Print and shaded views of the part. All mm, measured from the part's lowest x, y and z. Round coordinates to 2 decimals unless told otherwise and drop trailing zeros. Order: outer loops, then holes, each group sorted by start corner. A loop starts at its lowest first (then second) coordinate and runs counter-clockwise, first axis right, second up.
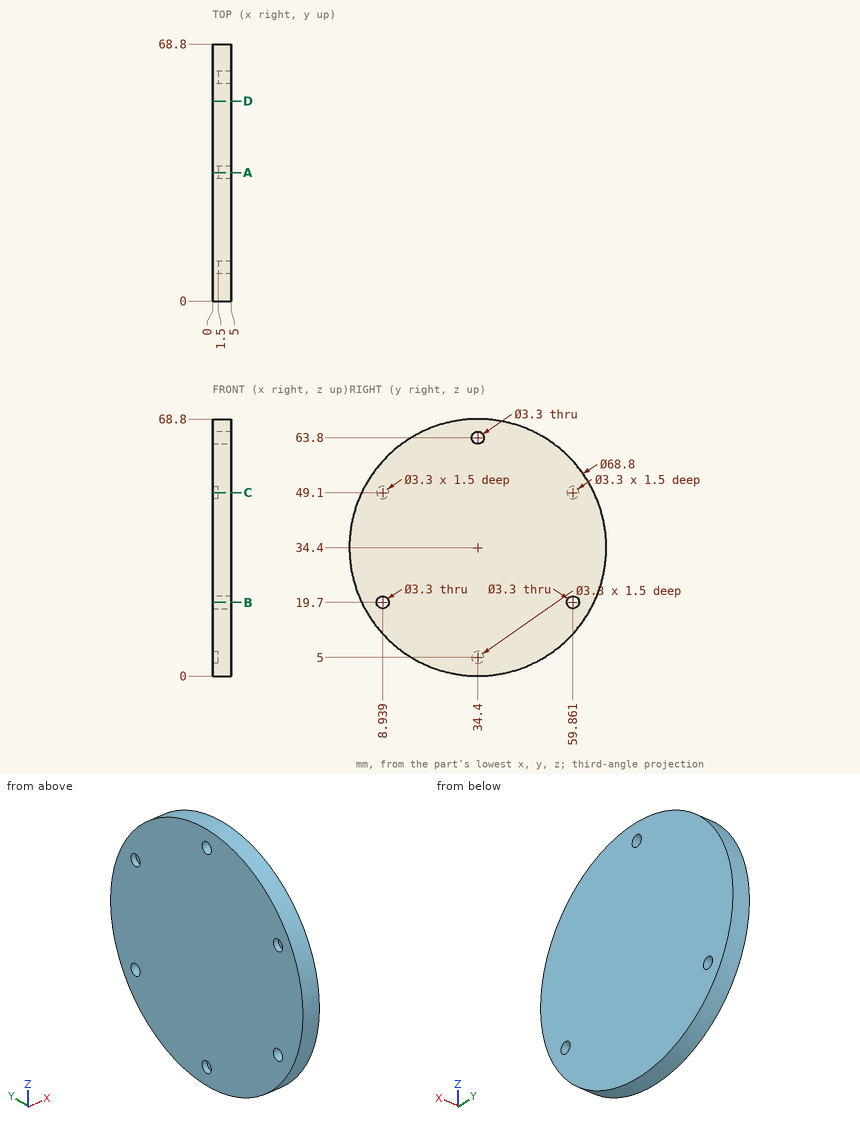
1. Pin check, flat tips, straight feed: P1, Ø1, axis at y = 9, z = 49, coming from the -X side; P2, Ø2, axis at x = 2.5, y = 56.5, coming from the -Z side; P3, Ø3, axis at x = 3, y = 31, coming from the +Z side. Stop position of each tip, or through.
2. Cut at B-B, the plane z = 19.7. Write the cut outline in (x, y), and give its area (3 significant figures).
3. Cut at A-A, the plane y = 34.4. Write the cut outline in (x, z).
4. Cut at C-C, the plane z = 49.1. Write the cut outline in (x, y).
5. Cut at D-D, the plane y = 53.5. Write the cut outline in (x, z).
6. Drill centre lines: line 1 (Y direction, x = 1.15, z = 49.1); line 2 (Y direction, x = 3.95, z = 64.5) (1 decimal); line 3 (Y direction, x = 4.7, z = 20.5). Where is each one in solid material? Low to high.
Outcome:
1. P1: stops at x = 1.5
1. P2: stops at z = 7.23
1. P3: stops at z = 68.75
2. outline: (0, 3.3) - (5, 3.3) - (5, 7.29) - (0, 7.29) - close; (0, 10.59) - (5, 10.59) - (5, 58.21) - (0, 58.21) - close; (0, 61.51) - (5, 61.51) - (5, 65.5) - (0, 65.5) - close
2. area: 278 mm2
3. outline: (0, 0) - (5, 0) - (5, 62.15) - (0, 62.15) - (0, 6.65) - (1.5, 6.65) - (1.5, 3.35) - (0, 3.35) - close; (0, 65.45) - (5, 65.45) - (5, 68.8) - (0, 68.8) - close
4. outline: (0, 3.3) - (5, 3.3) - (5, 65.5) - (0, 65.5) - (0, 61.51) - (1.5, 61.51) - (1.5, 58.21) - (0, 58.21) - (0, 10.59) - (1.5, 10.59) - (1.5, 7.29) - (0, 7.29) - close
5. outline: (0, 5.79) - (5, 5.79) - (5, 63.01) - (0, 63.01) - close
6. line 1: y = 3.3 to 7.29, 10.59 to 58.21, 61.51 to 65.5
6. line 2: y = 17.7 to 32.9, 35.9 to 51.1
6. line 3: y = 2.93 to 7.5, 10.38 to 58.42, 61.3 to 65.87
